Verification items for the finished model (mm, model axes). Give positions to 0.01 mm unless a question says otherwise; leave off trailing zeros. Write each loop counter-clockwise with the first axis right and the second up, starting at its lowest first coordinate (ties: lowest second). Pieces come first, ordered by that corner, then holes. Notation, with made-up numbers: (-34, -33) - (-29, -33) arc R20 cw to (-29, -8) - close; hole circle Ø5 at (-35, -30). An arc over 180 degrees is marked (long way). Answer as a JSON object with one key per item and string values. Group by question number.
Item 1: Sectioned sample at B-B, the plane x = -12. Record the boundary of the cut face in (y, z), and give its area (3 significant figures).
Item 2: Sectioned sample at C-C, the plane y = -17.25. Record the boundary of the cut face in (x, z) (1 decimal), and give its area (3 significant figures).
Item 3: Scan lines: line 1 along X through (y, z) = (-4.5, 25.5); line 2 along Z through (x, y) = (-1, -2.5); line 3 along Z through (x, y) = (-15.5, -14.5). Record each from-to range of solid material in increasing order. Write a range as [from, to].
Item 4: Go/stop test with a flat-tipped pin: pin 1 (1 mm diameter, centred on x = 9, y = -6, fed in from +Z). Record where the tip stops, or that it passes through.
Item 5: Sectioned sample at A-A, the plane z = 19.5. Record the boundary of the cut face in (x, y), and give its area (3 significant figures).
Item 6: Sectioned sample at D-D, the plane x = 7. Record the boundary of the cut face in (y, z).
```python
from build123d import *

# Parameters (mm, degrees)
F0_W     = 45
F0_H     = 60
F0_R     = 5
F1_DEPTH = 25


with BuildPart() as f1:
    # F0 (on Front) → F1 (new body)
    with BuildSketch(Plane.XZ):
        with BuildLine():
            ThreePointArc((22.5, 30), (0, 40), (-22.5, 30))
            Line((-22.5, 30), (22.5, 30))
        make_face()
        Rectangle(F0_W, F0_H)
        with Locations((-11.565693, 21.846309)):
            Circle(F0_R, mode=Mode.SUBTRACT)
        with Locations((10.13783, 21.560736)):
            Circle(F0_R, mode=Mode.SUBTRACT)
    extrude(amount=F1_DEPTH)


solid = f1.part
```
Geometry check:
{
 "1": {"outline": "(-25, -30) - (0, -30) - (0, 16.87) - (-25, 16.87) - close; (-25, 26.83) - (0, 26.83) - (0, 37.52) - (-25, 37.52) - close", "area": "1,440 mm^2"},
 "2": {"outline": "(-22.5, -30) - (22.5, -30) - (22.5, 30) arc R30.3 ccw to (-22.5, 30) - close; hole circle Ø10 at (-11.6, 21.8); hole circle Ø10 at (10.1, 21.6)", "area": "2,850 mm^2"},
 "3": {"line 1": "[-22.5, -14.98], [-8.15, 7.06], [13.22, 22.5]", "line 2": "[-30, 39.98]", "line 3": "[-30, 18.76], [24.93, 35.74]"},
 "4": {"pin 1": "z = 38.78"},
 "5": {"outline": "(-22.5, -25) - (-15.98, -25) - (-15.98, 0) - (-22.5, 0) - close; (-7.15, -25) - (5.58, -25) - (5.58, 0) - (-7.15, 0) - close; (14.69, -25) - (22.5, -25) - (22.5, 0) - (14.69, 0) - close", "area": "676 mm^2"},
 "6": {"outline": "(-25, -30) - (0, -30) - (0, 17.67) - (-25, 17.67) - close; (-25, 25.45) - (0, 25.45) - (0, 39.18) - (-25, 39.18) - close"}
}
